from build123d import *

# Parameters (mm, degrees)
F1_DEPTH = 15
F2_T     = -10
F3_R     = 4.99999
F5_R     = 15
F6_DEPTH = 25


# Not quite as in the source:
# - a fillet or chamfer is up to 0.001 mm smaller than in the source, because OpenCascade refuses the exact size


with BuildPart() as f1:
    # F0 (on Top) → F1 (new body)
    with BuildSketch(Plane.XY):
        Polygon((87.8512188792, -15.3126027435), (0, 0), (-120.9431961179, -4.3791108765), (-143.5155719519, -80.9135511518), (-68.7445923686, -112.6559451222), (62.802106142, -141.5623724461), (104.0751114488, -54.4615574181), align=None)
    extrude(amount=F1_DEPTH)

    # F2
    f2_openings = [f1.faces().sort_by_distance(p)[0] for p in [
        (-14.831711, -62.307507, 15),
    ]]
    offset(amount=F2_T, openings=f2_openings)

    # F3 (radius 5 in the source; OpenCascade refuses exactly that, so slightly less here)
    f3_edges = [f1.edges().sort_by_distance(p)[0] for p in [
        (-143.515572, -80.913551, 7.5),
        (-68.744592, -112.655945, 7.5),
        (62.802106, -141.562372, 7.5),
        (104.075111, -54.461557, 7.5),
        (87.851219, -15.312603, 7.5),
        (0, 0, 7.5),
        (-120.943196, -4.379111, 7.5),
        (75.155878, -92.138524, 10),
        (-4.258831, -116.587633, 10),
        (57.17386, -130.087018, 12.5),
        (-65.691523, -103.088247, 12.5),
        (-98.546913, -89.140205, 10),
        (86.927893, -39.205026, 10),
        (93.137896, -54.19003, 12.5),
        (80.717891, -24.220021, 12.5),
        (40.016406, -17.12569, 10),
        (-0.685079, -10.031358, 12.5),
        (-57.036491, -12.07173, 10),
        (-122.395103, -44.652133, 10),
        (-113.387903, -14.112102, 12.5),
        (-131.402304, -75.192163, 12.5),
    ]]
    fillet(f3_edges, radius=F3_R)

    # F4: F1 across plane


with BuildPart() as f1_1:
    add(f1.part)
    add(f1.part.mirror(Plane.XY))

    # F5 (on face) → F6 (cut)
    with BuildSketch(Plane.XY.offset(10)):
        with Locations((10.5543992388, -65)):
            Circle(F5_R)
    extrude(amount=-F6_DEPTH, mode=Mode.SUBTRACT)


solid = f1_1.part
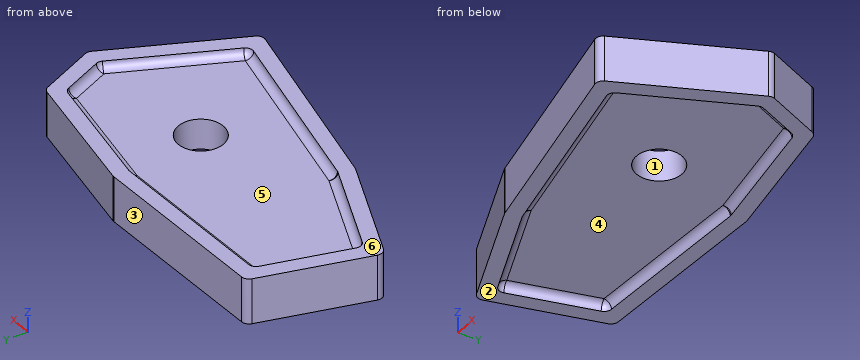
CAD build for the part. Positions are in the model's coordinates, mm. Face numbers are marked on the shaded views. A direction names the side the tool comes from. Round coordinates to 2 decimals unless told otherwise and drop trailing zeros. Write each loop counter-clockwise with the first axis right and the second up, starting at its lowest first coordinate (ties: lowest second). Pieces come first, ordered by that corner, then holes. Notation, with made-up numbers: M -0.5,43 L 40.5,43 A32 cw 40.5,70 Z; hole C -29,11.25 d8. An arc over 180 degrees is marked long. Use a Markdown table: item, result. Add a question column.
1. Flat gauge pins, fed straight in: P1, Ø6, axis at y = -71.5, z = 6.5, coming from the +X side; P2, Ø4, axis at x = 71, y = -41, coming from the +Z side; P3, Ø1.5, axis at x = -110, z = -11.5, coming from the +Y side. Where does each tip first touch, or does it go through?
2. Drill centre lines: probe 1 along Z at (x, y) = (15.5, -111.5); probe 2 along X at (y, z) = (-86.5, 4.25); probe 3 along Y at (x, z) = (20.5, -13.75). Where is each one in solid material? Low to high.
3. 3-axis set-ups, long thin cutter, end or side, ignore diameter. For the marked faces 4, 5 and 6: which of +Z, -Z, +X, -X, +Y, -Y reach the whole face in a straight line?
4. Pull direction Y, two halves, no side cores. Call the marked faces 1, 2 and 3: released by +Y, released by -Y, zero draft, split by the parting line, or undercut.
5. Slice it at B-B on z = 12.5. Give the cut face in (x, y) (3 decimals), then the cut area to 3 significant figures.
6. Slice it at A-A on z = -3. Give the cut face in (x, y).
Reply:
| question | item | result |
|---|---|---|
| 1 | P1 | stops at x = 97.42 |
| 1 | P2 | stops at z = 10 |
| 1 | P3 | stops at y = -3.96 |
| 2 | probe 1 | z = -10 to 10 |
| 2 | probe 2 | x = -130.36 to 88.89 |
| 2 | probe 3 | y = -132.27 to -121.87, -13.89 to -3.57 |
| 3 | face 4 | -Z |
| 3 | face 5 | +Z |
| 3 | face 6 | +Z, +X, -X, +Y, -Y |
| 4 | face 1 | undercut |
| 4 | face 2 | zero draft |
| 4 | face 3 | released by +Y |
| 5 | outline | M -142.255,-76.638 A5 ccw -139.413,-82.655 L -69.172,-112.475 A5 ccw -68.291,-112.756 L 58.915,-140.708 A5 ccw 64.506,-137.966 L 103.125,-56.467 A5 ccw 103.226,-52.412 L 88.904,-17.852 A5 ccw 85.143,-14.841 L 0.516,-0.09 A5 ccw -0.523,-0.019 L -117.346,-4.249 A5 ccw -121.961,-7.831 Z; hole M -129.499,-71.107 A4.33 ccw -127.038,-76.317 L -65.857,-102.29 A4.33 ccw -65.094,-102.534 L 53.43,-128.579 A4.33 ccw 58.273,-126.204 L 91.582,-55.908 A4.33 ccw 91.67,-52.397 L 81.151,-27.016 A4.33 ccw 77.895,-24.408 L -0.284,-10.781 A4.33 ccw -1.184,-10.72 L -109.767,-14.651 A4.33 ccw -113.764,-17.754 Z |
| 5 | area | 6,470 mm^2 |
| 6 | outline | M -142.25,-76.64 A5 ccw -139.41,-82.66 L -69.17,-112.47 A5 ccw -68.29,-112.76 L 58.91,-140.71 A5 ccw 64.51,-137.97 L 103.12,-56.47 A5 ccw 103.23,-52.41 L 88.9,-17.85 A5 ccw 85.14,-14.84 L 0.52,-0.09 A5 ccw -0.52,-0.02 L -117.35,-4.25 A5 ccw -121.96,-7.83 Z; hole C 10.55,-65 d30 |
